Autodesk Inventor part; units mm, degrees
ref_plane "YZ Plane" through (0, 0, 0) normal (1, 0, 0) x (0, 1, 0)
ref_plane "XZ Plane" through (0, 0, 0) normal (0, 1, 0) x (-1, 0, 0)
ref_plane "XY Plane" through (0, 0, 0) normal (0, 0, 1) x (1, 0, 0)
ref_plane "Work Plane1" through (52.5141, 202.7033, 6.4479) normal (0, 0, -1) x (0, 1, 0)
sketch "Sketch1" plane through (52.5141, 202.7033, 6.4479) normal (0, 0, -1) x (0, 1, 0)
  circle A0 centre (-59.8114, -30.5) radius 1.4 construction
  circle A1 centre (-38.8114, -18.3756) radius 1.4
  circle A2 centre (-38.8114, -42.6244) radius 1.4 construction
  circle A3 centre (41, 0) radius 1.65
  circle A4 centre (-9, 0) radius 1.65
  circle A5 centre (-9, 50) radius 1.65
  circle A6 centre (41, 50) radius 1.65
  circle A7 centre (16, 50) radius 1.65
  circle A8 centre (-9, 25) radius 1.65
  circle A9 centre (16, 0) radius 1.65
  circle A10 centre (41, 25) radius 1.65
  line L0 (80, 55) -> (-80, 55)
  line L1 (-80, 55) -> (-80, -55)
  line L2 (-80, -55) -> (80, -55)
  line L3 (80, -55) -> (80, 55)
  line L4 (-36.5, 0) -> (-36.5, -50)
  line L5 (-14, 0) -> (-36.5, 0)
  line L6 (-14, -5) -> (-14, 0)
  line L7 (72, -5) -> (-14, -5)
  line L8 (72, -50) -> (72, -5)
  line L9 (-36.5, -50) -> (72, -50)
  line L10 (-4, 45) -> (-4, 5)
  line L11 (36, 45) -> (-4, 45)
  line L12 (36, 5) -> (36, 45)
  line L13 (-4, 5) -> (36, 5)
  line L14 (-64.5989, -17.0433) -> (-64.5989, -57.0433) construction
  line L15 (-64.5989, -57.0433) -> (-34.5989, -57.0433) construction
  line L16 (-34.5989, -57.0433) -> (-34.5989, -17.0433) construction
  line L17 (-34.5989, -17.0433) -> (-64.5989, -17.0433) construction
  line L18 (-34.8114, -13.0433) -> (-63.8114, -13.0433)
  line L19 (-63.8114, -13.0433) -> (-63.8114, -52.6244)
  line L20 (-63.8114, -52.6244) -> (-34.8114, -52.6244)
  line L21 (-34.8114, -52.6244) -> (-34.8114, -13.0433)
  circle A11 centre (-59.8114, -30.5) radius 2.95
  circle A12 centre (-38.8114, -18.3756) radius 2.95
  circle A13 centre (-38.8114, -42.6244) radius 2.95 construction
  line L22 (-36.5, -35.1157) -> (-41.75, -35.1157) construction
  line L23 (-41.75, -35.1157) -> (-41.75, -38.5657) construction
  line L24 (-41.75, -38.5657) -> (-56.86, -38.5657) construction
  line L25 (-56.86, -38.5657) -> (-56.86, -35.1157) construction
  line L26 (-56.86, -35.1157) -> (-60.26, -35.1157) construction
  line L27 (-60.26, -35.1157) -> (-60.26, -52.0657) construction
  line L28 (-60.26, -52.0657) -> (-36.5, -52.0657) construction
  line L29 (-36.5, -52.0657) -> (-36.5, -35.1157) construction
  line L30 (-41.75, -28.3657) -> (-36.5, -28.3657) construction
  line L31 (-36.5, -28.3657) -> (-36.5, -25.0657) construction
  line L32 (-36.5, -25.0657) -> (-60.26, -25.0657) construction
  line L33 (-60.26, -25.0657) -> (-60.26, -28.3657) construction
  line L34 (-60.26, -28.3657) -> (-56.86, -28.3657) construction
  line L35 (-56.86, -28.3657) -> (-56.86, -27.0942) construction
  line L36 (-56.86, -27.0942) -> (-41.75, -27.0942) construction
  line L37 (-41.75, -27.0942) -> (-41.75, -28.3657) construction
  line L38 (-56.86, -35.1157) -> (-60.26, -35.1157) construction
  line L39 (-56.86, -38.5657) -> (-56.86, -35.1157) construction
  line L40 (-41.75, -38.5657) -> (-56.86, -38.5657) construction
  line L41 (-41.75, -35.1157) -> (-41.75, -38.5657) construction
  line L42 (-36.5, -35.1157) -> (-41.75, -35.1157) construction
  line L43 (-36.5, -35.05) -> (-36.5, -35.1157) construction
  line L44 (-36.5, -35.05) -> (-56.86, -35.05) construction
  line L45 (-36.5, -34.78) -> (-36.5, -35.05) construction
  line L46 (-36.5, -34.78) -> (-56.86, -34.78) construction
  line L47 (-36.5, -34.51) -> (-36.5, -34.78) construction
  line L48 (-36.5, -34.51) -> (-56.86, -34.51) construction
  line L49 (-36.5, -34.24) -> (-36.5, -34.51) construction
  line L50 (-36.5, -34.24) -> (-56.86, -34.24) construction
  line L51 (-36.5, -33.97) -> (-36.5, -34.24) construction
  line L52 (-36.5, -33.97) -> (-56.86, -33.97) construction
  line L53 (-36.5, -33.7) -> (-36.5, -33.97) construction
  line L54 (-36.5, -33.7) -> (-56.86, -33.7) construction
  line L55 (-36.5, -33.43) -> (-36.5, -33.7) construction
  line L56 (-36.5, -33.43) -> (-56.86, -33.43) construction
  line L57 (-36.5, -33.16) -> (-36.5, -33.43) construction
  line L58 (-36.5, -33.16) -> (-56.86, -33.16) construction
  line L59 (-36.5, -32.89) -> (-36.5, -33.16) construction
  line L60 (-36.5, -32.89) -> (-56.86, -32.89) construction
  line L61 (-36.5, -32.62) -> (-36.5, -32.89) construction
  line L62 (-36.5, -32.62) -> (-56.86, -32.62) construction
  line L63 (-36.5, -32.35) -> (-36.5, -32.62) construction
  line L64 (-36.5, -32.35) -> (-56.86, -32.35) construction
  line L65 (-36.5, -32.08) -> (-36.5, -32.35) construction
  line L66 (-36.5, -32.08) -> (-56.86, -32.08) construction
  line L67 (-36.5, -31.81) -> (-36.5, -32.08) construction
  line L68 (-36.5, -31.81) -> (-56.86, -31.81) construction
  line L69 (-36.5, -31.54) -> (-36.5, -31.81) construction
  line L70 (-36.5, -31.54) -> (-56.86, -31.54) construction
  line L71 (-36.5, -31.27) -> (-36.5, -31.54) construction
  line L72 (-36.5, -31.27) -> (-56.86, -31.27) construction
  line L73 (-36.5, -31) -> (-36.5, -31.27) construction
  line L74 (-36.5, -31) -> (-56.86, -31) construction
  line L75 (-36.5, -30.73) -> (-36.5, -31) construction
  line L76 (-36.5, -30.73) -> (-56.86, -30.73) construction
  line L77 (-36.5, -30.46) -> (-36.5, -30.73) construction
  line L78 (-36.5, -30.46) -> (-56.86, -30.46) construction
  line L79 (-36.5, -30.19) -> (-36.5, -30.46) construction
  line L80 (-36.5, -30.19) -> (-56.86, -30.19) construction
  line L81 (-36.5, -29.92) -> (-36.5, -30.19) construction
  line L82 (-36.5, -29.92) -> (-56.86, -29.92) construction
  line L83 (-36.5, -29.65) -> (-36.5, -29.92) construction
  line L84 (-36.5, -29.65) -> (-56.86, -29.65) construction
  line L85 (-36.5, -29.38) -> (-36.5, -29.65) construction
  line L86 (-36.5, -29.38) -> (-56.86, -29.38) construction
  line L87 (-36.5, -29.11) -> (-36.5, -29.38) construction
  line L88 (-36.5, -29.11) -> (-56.86, -29.11) construction
  line L89 (-36.5, -28.84) -> (-36.5, -29.11) construction
  line L90 (-36.5, -28.84) -> (-56.86, -28.84) construction
  line L91 (-36.5, -28.3657) -> (-36.5, -28.84) construction
  line L92 (-41.75, -28.3657) -> (-36.5, -28.3657) construction
  line L93 (-41.75, -27.0942) -> (-41.75, -28.3657) construction
  line L94 (-56.86, -27.0942) -> (-41.75, -27.0942) construction
  line L95 (-56.86, -28.3657) -> (-56.86, -27.0942) construction
  line L96 (-60.26, -28.3657) -> (-56.86, -28.3657) construction
  line L97 (-60.26, -35.1157) -> (-60.26, -28.3657) construction
  line L98 (-60.26, -25.0657) -> (-36.5, -25.0657) construction
  line L99 (-36.5, -25.0657) -> (-36.5, -52.0657) construction
  line L100 (-60.26, -52.0657) -> (-60.26, -25.0657) construction
  line L101 (-57.1632, -22.5233) -> (-33.4032, -22.5233) construction
  line L102 (-33.4032, -22.5233) -> (-33.4032, -49.5233) construction
  line L103 (-33.4032, -49.5233) -> (-57.1632, -49.5233) construction
  line L104 (-57.1632, -49.5233) -> (-57.1632, -22.5233) construction
  circle A14 centre (-38.8114, -42.6244) radius 2.95
  point P0 (-202.7033, -52.5141)
  point P1 (-56.7146, -27.9576)
  dimension "d0" = 4
  dimension "d2" = 4
  dimension "d3" = 4
  dimension "d4" = 5.9
  dimension "d5" = 5.9
  dimension "d6" = 5.9
  dimension "d10" = 10
extrude "Extrusion1" add sketch "Sketch1" along normal blind 4 contours L18 L21 L9 L4 A14 A12 | L4 A12 A14 L9 L21 L20 L19 L18
sketch "Sketch2" plane through (52.5141, 202.7033, 2.4479) normal (0, 0, -1) x (-1, 0, 0)
  circle A0 centre (42.6244, -38.8114) radius 2.95
  circle A1 centre (18.3756, -38.8114) radius 2.95
  circle A2 centre (30.5, -59.8114) radius 2.95
  line L0 (13.0433, -34.8114) -> (13.0433, -63.8114)
  line L1 (13.0433, -63.8114) -> (52.6244, -63.8114)
  line L2 (52.6244, -63.8114) -> (52.6244, -34.8114)
  line L3 (52.6244, -34.8114) -> (13.0433, -34.8114)
  point P0 (52.5141, -202.7033)
extrude "Extrusion2" add sketch "Sketch2" along normal blind 1.5 contours A0 | A1 | A2 | L3 L2 L1 L0
sketch "Sketch6" plane through (52.5141, 202.7033, 0.9479) normal (0, 0, -1) x (-1, 0, 0)
  line L0 (13.0433, -34.8114) -> (13.0433, -63.8114)
  line L1 (13.0433, -63.8114) -> (52.6244, -63.8114)
  line L2 (52.6244, -63.8114) -> (52.6244, -34.8114)
  line L3 (52.6244, -34.8114) -> (13.0433, -34.8114)
  circle A0 centre (42.6244, -38.8114) radius 2.95
  circle A1 centre (18.3756, -38.8114) radius 2.95
  circle A2 centre (30.5, -59.8114) radius 2.95
  line L4 (3.3756, -34.8114) -> (57.6244, -34.8114)
  line L5 (57.6244, -34.8114) -> (57.6244, -74.8114)
  line L6 (57.6244, -74.8114) -> (3.3756, -74.8114)
  line L7 (3.3756, -74.8114) -> (3.3756, -34.8114)
  point P0 (52.5141, -202.7033)
  dimension "d34" = 15
  dimension "d35" = 15
  dimension "d36" = 15
extrude "Extrusion6" add sketch "Sketch6" against normal up to surface (5.5 mm away) contours L0 L1 L2 L4 L5 L6 L7
sketch "Sketch7" plane through (52.5141, 202.7033, 0.9479) normal (0, 0, -1) x (-1, 0, 0)
  circle A0 centre (30.5, -59.8114) radius 2.95
  circle A1 centre (18.3756, -38.8114) radius 2.95
  circle A2 centre (42.6244, -38.8114) radius 2.95
  line L0 (30.5, -59.8114) -> (42.6244, -38.8114)
  line L1 (42.6244, -38.8114) -> (18.3756, -38.8114)
  line L2 (18.3756, -38.8114) -> (30.5, -59.8114)
  circle A3 centre (30.5, -45.8114) radius 7
  circle A4 centre (30.5, -45.8114) radius 6.2512
  point P0 (52.5141, -202.7033)
extrude "Extrusion7" cut sketch "Sketch7" against normal through all contours A3 | A4
fillet "Fillet1" radius 4 4 edges at (49.1384, 127.8919, 3.6979) (49.1384, 167.8919, 3.6979) (-5.1103, 127.8919, 3.6979) (-5.1103, 167.8919, 3.6979)
sketch "Sketch8" plane through (52.5141, 202.7033, 0.9479) normal (0, 0, -1) x (-1, 0, 0)
  circle A0 centre (51.3406, -45.4668) radius 1.6
  circle A1 centre (11.3406, -45.4668) radius 1.6
  arc A2 (57.6244, -38.8114) -> (53.6244, -34.8114) centre (53.6244, -38.8114) ccw
  line L0 (7.3756, -34.8114) -> (53.6244, -34.8114)
  arc A3 (7.3756, -34.8114) -> (3.3756, -38.8114) centre (7.3756, -38.8114) ccw
  line L1 (3.3756, -70.8114) -> (3.3756, -38.8114)
  arc A4 (3.3756, -70.8114) -> (7.3756, -74.8114) centre (7.3756, -70.8114) ccw
  line L2 (53.6244, -74.8114) -> (7.3756, -74.8114)
  arc A5 (53.6244, -74.8114) -> (57.6244, -70.8114) centre (53.6244, -70.8114) ccw
  line L3 (57.6244, -38.8114) -> (57.6244, -70.8114)
  circle A6 centre (31.3406, -58.6258) radius 1.6
  point P0 (52.5141, -202.7033)
hole "Hole1" at (1.1735, 157.2365, 0.9479) at (21.1735, 144.0776, 0.9479) at (41.1735, 157.2365, 0.9479) direction (0, 0, 1) diameter 2.8 end through all
properties part number "cellSTORM_v5_chiptray_new_25.4mm_0"
Part model, mm, in its own coordinate system. A direction names the side the tool comes from. Coordinates: 2 decimals unless noted, no trailing zeros. Order: outer loops, then holes, each group sorted by start corner. A loop starts at its lowest first (then second) coordinate and runs counter-clockwise, first axis right, second up. Notation, with made-up numbers: (-1, -18.75) - (29, -18.75) arc R20 ccw to (29, 6.25) - close; hole circle Ø6 at (21.5, -30). An arc over 180 degrees is marked (long way). Return JSON: item names as keys, results as strings. Group by question number.
Item 1: Pull direction X, two halves, no side cores. Call faces 1 (the face through (41.71, 158.53, 3.74)), 2 (the face through (49.138, 148, 4)), 3 (the face through (22, 148, 0.948)): pulls with the +X half, pulls with the -X half, needs draft (parallel to the pull), parting line crosses it, or undercut.
Item 2: Drill centre lines: probe 1 along Y at (x, z) = (12, 4.2); probe 2 along X at (y, z) = (162, 5.15); probe 3 along X at (y, z) = (159.5, 1.6). Where is each one in solid material? Low to high. Write a range as from..to.
Item 3: Cut at C-C (y = 154.5). List the corners of the cut face in (x, z).
Item 4: Cut at B-B (z = 5.7). List the corners of the cut face in (x, y), plus the area to 3 significant figures.
Item 5: Cut at D-D (x = 35.5). List the corners of the cut face in (y, z), plus the area to 3 significant figures.
Item 6: Pin check, flat tip, straight feed: pin 1 (2 mm diameter, centred on x = 21.17, y = 144.08, fed in from +Z). Stop position of the tip, or through.
Item 7: Cut at A-A (x = 42). List the corners of the cut face in (y, z).
Item 8: Which spindle directions (+Z, -Z, +X, -X, +Y, -Y) get a long thin tool onto all of the face, cutting with end or side? Do faces 4 (the face through (1.71, 158.53, 3.74)), 5 (the face through (10, 164, 2.448)). Say none if no direction does.
Check values:
{
 "1": {"face 1": "undercut", "face 2": "pulls with the +X half", "face 3": "needs draft"},
 "2": {"probe 1": "y = 127.89..161.83, 165.95..167.89", "probe 2": "x = -5.11..7.63, 12.15..17.23, 26.8..31.88, 36.4..49.14", "probe 3": "x = -5.11..15.52, 28.51..49.14"},
 "3": {"outline": "(-5.11, 0.95) - (15.44, 0.95) - (15.44, 6.45) - (-5.11, 6.45) - close; (28.59, 0.95) - (49.14, 0.95) - (49.14, 6.45) - (28.59, 6.45) - close"},
 "4": {"outline": "(-5.11, 131.89) arc R4 ccw to (-1.11, 127.89) - (45.14, 127.89) arc R4 ccw to (49.14, 131.89) - (49.14, 163.89) arc R4 ccw to (45.14, 167.89) - (-1.11, 167.89) arc R4 ccw to (-5.11, 163.89) - close; hole circle Ø2.8 at (1.17, 157.24); hole circle Ø5.9 at (9.89, 163.89); hole circle Ø14 at (22.01, 156.89); hole circle Ø5.9 at (22.01, 142.89); hole circle Ø5.9 at (34.14, 163.89); hole circle Ø2.8 at (41.17, 157.24)", "area": "1,910 mm2"},
 "5": {"outline": "(127.89, 0.95) - (167.89, 0.95) - (167.89, 6.45) - (166.51, 6.45) - (166.51, 2.45) - (161.27, 2.45) - (161.27, 6.45) - (127.89, 6.45) - close", "area": "199 mm2"},
 "6": {"pin 1": "passes through"},
 "7": {"outline": "(127.89, 0.95) - (156.11, 0.95) - (156.11, 6.45) - (127.89, 6.45) - close; (158.37, 0.95) - (167.89, 0.95) - (167.89, 6.45) - (158.37, 6.45) - close"},
 "8": {"face 4": "+Z, -Z", "face 5": "+Z"}
}
